Geometry: final body of the model. Coordinates: model frame, mm. A direction names the side the tool comes from. Round coordinates to 2 decimals unless told otherwise and drop trailing zeros. Loops run counter-clockwise (first coordinate to the right, second up) from the corner with the lowest first, then second, coordinate; pieces in that order, holes last. Notation, with made-up numbers: (9, -36.5) - (45, -36.5) arc R30 cw to (45, 0.5) - close; hole circle Ø7 at (-9.75, 21.25). An arc over 180 degrees is marked (long way). Use CSV: the item, a comma, the result in double quotes.
Autodesk Inventor part; units mm, degrees
ref_plane "YZ Plane" through (0, 0, 0) normal (1, 0, 0) x (0, 1, 0)
ref_plane "XZ Plane" through (0, 0, 0) normal (0, 1, 0) x (-1, 0, 0)
ref_plane "XY Plane" through (0, 0, 0) normal (0, 0, 1) x (1, 0, 0)
sketch "Sketch1" plane through (0, 0, 0) normal (0, 0, 1) x (1, 0, 0)
  line L0 (-35.5, 13.25) -> (35.5, 13.25)
  line L1 (35.5, 13.25) -> (35.5, -13.25)
  line L2 (35.5, -13.25) -> (-35.5, -13.25)
  line L3 (-35.5, -13.25) -> (-35.5, 13.25)
  line L4 (-34.3, 12.05) -> (34.3, 12.05)
  line L5 (34.3, 12.05) -> (34.3, -12.05)
  line L6 (34.3, -12.05) -> (-34.3, -12.05)
  line L7 (-34.3, -12.05) -> (-34.3, 12.05)
  point P0 (0, 0)
  dimension "d0" = 71
  dimension "d1" = 26.5
  dimension "d2" = 35.5
  dimension "d3" = 13.25
  dimension "d4" = 1.2
  dimension "d5" = 1.2
  dimension "d6" = 1.2
  dimension "d7" = 1.2
extrude "Extrusion1" add sketch "Sketch1" along normal blind 100
fillet "Fillet1" radius 2 4 edges at (-34.3, 12.05, 50) (34.3, 12.05, 50) (34.3, -12.05, 50) (-34.3, -12.05, 50)
fillet "Fillet2" radius 3.25 4 edges at (-35.5, 13.25, 50) (-35.5, -13.25, 50) (35.5, -13.25, 50) (35.5, 13.25, 50)
sketch "Sketch2" plane through (0, 0, 100) normal (0, 0, 1) x (1, 0, 0)
  line L0 (-34.3, -10.05) -> (-34.3, 10.05)
  line L1 (-34.3, -7.9) -> (-31.3, -7.9)
  line L2 (-31.3, -7.9) -> (-31.3, -9.4)
  line L3 (-31.3, -9.4) -> (-34.3, -9.4)
  line L4 (-34.3, -9.4) -> (-34.3, -7.9)
  line L5 (34.3, 10.05) -> (34.3, -10.05)
  line L6 (34.3, -7.9) -> (31.3, -7.9)
  line L7 (31.3, -7.9) -> (31.3, -9.4)
  line L8 (31.3, -9.4) -> (34.3, -9.4)
  line L9 (34.3, -9.4) -> (34.3, -7.9)
  line L10 (-32.25, -13.25) -> (32.25, -13.25)
  line L11 (-34.3, -6.05) -> (-31.3, -6.05)
  line L12 (-31.3, -6.05) -> (-31.3, -4.55)
  line L13 (-31.3, -4.55) -> (-34.3, -4.55)
  line L14 (-34.3, -4.55) -> (-34.3, -6.05)
  line L15 (31.3, -6.05) -> (34.3, -6.05)
  line L16 (34.3, -6.05) -> (34.3, -4.55)
  line L17 (34.3, -4.55) -> (31.3, -4.55)
  line L18 (31.3, -4.55) -> (31.3, -6.05)
  point P0 (0, 0)
  dimension "d12" = 3.85
  dimension "d13" = 1.5
  dimension "d14" = 3
  dimension "d15" = 3
  dimension "d16" = 1.5
  dimension "d17" = 1.85
extrude "Extrusion2" add sketch "Sketch2" against normal blind 100
fillet "Fillet3" radius 1 4 edges at (-34.3, -4.55, 50) (-34.3, -9.4, 50) (34.3, -9.4, 50) (34.3, -4.55, 50)
sketch "Sketch3" plane through (0, 0, 100) normal (0, 0, 1) x (1, 0, 0)
  line L0 (32.25, 13.25) -> (-32.25, 13.25)
  line L1 (-35.5, 10) -> (-35.5, -10)
  line L2 (-32.25, -13.25) -> (32.25, -13.25)
  line L3 (35.5, -10) -> (35.5, 10)
  circle A0 centre (-32.5, 10.25) radius 2
  circle A1 centre (-32.5, -10.25) radius 2
  circle A2 centre (32.5, -10.25) radius 2
  circle A3 centre (32.5, 10.25) radius 2
  point P0 (0, 0)
  dimension "d21" = 3
  dimension "d22" = 3
  dimension "d23" = 3
  dimension "d24" = 3
  dimension "d25" = 3
  dimension "d26" = 3
  dimension "d27" = 3
  dimension "d28" = 3
  dimension "d29" = 4
  dimension "d30" = 4
  dimension "d31" = 4
  dimension "d32" = 4
extrude "Extrusion3" add sketch "Sketch3" against normal blind 100
sketch "Sketch4" plane through (0, 0, 100) normal (0, 0, 1) x (1, 0, 0)
  arc A0 (-34.3, 9.3782) -> (-31.6282, 12.05) centre (-32.5, 10.25) ccw
  arc A1 (31.6282, 12.05) -> (34.3, 9.3782) centre (32.5, 10.25) ccw
  arc A2 (31.3, -8.65) -> (31.6282, -12.05) centre (32.5, -10.25) ccw
  arc A3 (-31.6282, -12.05) -> (-31.3, -8.65) centre (-32.5, -10.25) ccw
  circle A4 centre (-32.5, 10.25) radius 1
  circle A5 centre (-32.5, -10.25) radius 1
  circle A6 centre (32.5, 10.25) radius 1
  circle A7 centre (32.5, -10.25) radius 1
  point P0 (0, 0)
  dimension "d35" = 2
  dimension "d36" = 2
  dimension "d37" = 2
  dimension "d38" = 2
extrude "Extrusion4" cut sketch "Sketch4" against normal blind 100
sketch "Sketch5" plane through (35.5, -10, 0) normal (1, 0, 0) x (0, 0, -1)
  line L0 (-100, 20) -> (-100, 0)
  line L1 (-100, 17) -> (-75, 17)
  line L2 (-75, 17) -> (-75, 14.9)
  line L3 (-75, 14.9) -> (-100, 14.9)
  line L4 (-100, 14.9) -> (-100, 17)
  line L5 (-100, 20) -> (0, 20)
  point P0 (0, 10)
  dimension "d41" = 2.1
  dimension "d42" = 3
  dimension "d43" = 25
extrude "Extrusion5" cut sketch "Sketch5" against normal blind 2
sketch "Sketch6" plane through (0, 0, 100) normal (0, 0, 1) x (1, 0, 0)
  line L0 (34.3, -6.05) -> (34.3, -7.9)
  line L1 (-34.3, -7.9) -> (-34.3, -6.05)
  line L2 (-31.3, -7.9) -> (-34.3, -7.9)
  line L3 (-31.3, -7.9) -> (-29.5, -7.9)
  line L4 (-29.5, -7.9) -> (-29.5, -9.4)
  line L5 (-29.5, -9.4) -> (-31.3, -9.4)
  line L6 (-31.3, -9.4) -> (-31.3, -7.9)
  line L7 (-31.3, -6.05) -> (-31.3, -4.55)
  line L8 (-31.3, -4.55) -> (-29.5, -4.55)
  line L9 (-29.5, -4.55) -> (-29.5, -6.05)
  line L10 (-29.5, -6.05) -> (-31.3, -6.05)
  line L11 (-31.3, -6.05) -> (-31.3, -4.55)
  line L12 (31.3, -4.55) -> (29.5, -4.55)
  line L13 (29.5, -4.55) -> (29.5, -6.05)
  line L14 (29.5, -6.05) -> (31.3, -6.05)
  line L15 (31.3, -6.05) -> (31.3, -4.55)
  line L16 (31.3, -7.9) -> (29.5, -7.9)
  line L17 (29.5, -7.9) -> (29.5, -9.4)
  line L18 (29.5, -9.4) -> (31.3, -9.4)
  line L19 (31.3, -9.4) -> (31.3, -7.9)
  line L20 (-31.3, -6.05) -> (-34.3, -6.05)
  line L21 (-34.3, -6.05) -> (-32.5, -6.05)
  line L22 (-32.5, -6.05) -> (-32.5, -7.9)
  line L23 (-32.5, -7.9) -> (-34.3, -7.9)
  line L24 (-34.3, -7.9) -> (-34.3, -6.05)
  line L25 (34.3, -6.05) -> (31.3, -6.05)
  line L26 (31.3, -7.9) -> (34.3, -7.9)
  line L27 (34.3, -6.05) -> (32.5, -6.05)
  line L28 (32.5, -6.05) -> (32.5, -7.9)
  line L29 (32.5, -7.9) -> (34.3, -7.9)
  line L30 (34.3, -7.9) -> (34.3, -6.05)
  point P0 (0, 0)
  dimension "d46" = 68.6
  dimension "d47" = 65
  dimension "d48" = 1.8
  dimension "d49" = 1.8
  dimension "d50" = 3
  dimension "d51" = 1.5
  dimension "d52" = 3
extrude "Extrusion6" add sketch "Sketch6" against normal blind 100
sketch "Sketch7" plane through (0, 0, 100) normal (0, 0, 1) x (1, 0, 0)
  line L0 (-32.25, -13.25) -> (32.25, -13.25)
  line L1 (32.25, 13.25) -> (-32.25, 13.25)
  line L2 (35.5, -10) -> (35.5, 4.9)
  line L3 (-35.5, 10) -> (-35.5, -10)
  point P0 (0, 0)
  dimension "d55" = 26.5
  dimension "d56" = 71
properties part number "case"
Item 1: Section B-B on z = 28. Give the number of separate pieces and of enclosed holes in the cut face, plus the area to 3 significant figures.
Final values:
separate pieces,"1"
enclosed holes,"5"
area,"286 mm²"
Item 2: Pin query (flat end, axial travel): P1, Ø1, axis at x = 35, y = 6, coming from the +Z side. Return the tip coordinate at first contact, or that it passes through.
Final values:
P1,"stops at z = 75"
Item 3: Mould query, pull axis X, two halves, no side actions, for faces 1 (the cylindrical face through (-33.237, 10.926, 50.7)), 2 (the flat face through (-3, -13, 100)), 3 (the flat face through (-35.5, 0, 49)), 4 (the flat face through (34.3, 3, 49)). Classes: released by +X, released by -X, zero draft, split by the parting line, or undercut.
Final values:
face 1,"undercut"
face 2,"zero draft"
face 3,"released by -X"
face 4,"undercut"
Item 4: Section A-A on x = 16. Return the cut outline in (y, z), plus the area to 3 significant figures.
Final values:
outline,"(-13.25, 0) - (-12.05, 0) - (-12.05, 100) - (-13.25, 100) - close; (12.05, 0) - (13.25, 0) - (13.25, 100) - (12.05, 100) - close"
area,"240 mm²"
Item 5: Material intervals for line 1 (X direction, y = -0.75, z = 40.5); line 2 (Y direction, x = 21, z = 73); line 3 (X direction, y = -5.25, z = 16), sorted ascending.
Final values:
line 1,"x = -35.5 to -34.3, 34.3 to 35.5"
line 2,"y = -13.25 to -12.05, 12.05 to 13.25"
line 3,"x = -35.5 to -29.5, 29.5 to 35.5"
Item 6: Reachability of faces 5 (the flat face through (0, -13.25, 49)), 6 (the flat face through (0, 12.05, 49)) from +Z, -Z, +X, -X, +Y, -Y: full face, straight path, thin tool, end or side. Return the list, or none.
Final values:
face 5,"+Z, -Z, +X, -X, -Y"
face 6,"+Z, -Z"
